Part model, mm, in its own coordinate system. A direction names the side the tool comes from. Round coordinates to 2 decimals unless told otherwise and drop trailing zeros. Loops run counter-clockwise (first coordinate to the right, second up) from the corner with the lowest first, then second, coordinate; pieces in that order, holes last.
Autodesk Inventor part; units mm, degrees
ref_plane "Start Plane" through (0, 0, 0) normal (1, 0, 0) x (0, 1, 0)
ref_plane "XZ Plane" through (0, 0, 0) normal (0, 1, 0) x (-1, 0, 0)
ref_plane "XY Plane" through (0, 0, 0) normal (0, 0, 1) x (1, 0, 0)
sketch "Main Sketch" plane through (0, 0, 0) normal (0, 0, 1) x (1, 0, 0)
  line L0 (0, 0) -> (210, 0)
  line L1 (0, 0) -> (0, 15)
  line L2 (0, 15) -> (40, 15)
  line L3 (40, 15) -> (40, 20)
  line L4 (90, 20) -> (90, 15)
  line L5 (40, 20) -> (90, 20)
  line L6 (210, 15) -> (210, 0)
  line L7 (90, 15) -> (210, 15)
  dimension "d3" = 30
  dimension "d4" = 40
  dimension "d5" = 30
revolve "Revolution1" add sketch "Main Sketch" angle 360 about axis through (0, 0, 0) along (1, 0, 0)
chamfer "Chamfer3" distance 2 angle 45 1 edges at (40, -15, 0) measured on face at (26.6667, 14.8058, -2.4062)
chamfer "Chamfer1" distance 0.5 angle 45 1 edges at (0, -15, 0) measured on face at (25.3333, 14.9514, -1.207)
chamfer "Chamfer2" distance 2 angle 45 1 edges at (90, -15, 0) measured on face at (170, 14.9514, -1.207)
equation "\"Length\" = 210"
properties part number "Shaft" material "Steel"
1) Slice it at C-C, the plane x = 53.5. Give the cut face in (y, z).
Values:
outline: circle Ø40 at (0, 0)
2) Tool access for faces 1 (the face through (40, -9, -15)), 2 (the face through (210, 0, 0)), 3 (the face through (90, -9, -15)): list every direction of +Z, -Z, +X, -X, +Y, -Y with a clear straight run to the whole face (end or side of a thin tool).
Values:
face 1: -X
face 2: +Z, -Z, +X, +Y, -Y
face 3: +X
3) Wall check: line 1 along Y through (x, z) = (83, 1); line 2 along X through (y, z) = (-8.5, -18); line 3 along Y through (x, z) = (177.5, -0.5). Give the ranges that are in metal, low to high.
Values:
line 1: y = -19.97 to 19.97
line 2: x = 40 to 90
line 3: y = -14.99 to 14.99
4) Slice it at B-B, the plane x = 96.5. Give the cut face in (y, z).
Values:
outline: circle Ø30 at (0, 0)
5) Drop flat-ended pins along their axis: pin 1 Ø12 at (x, z) = (84.5, -12) entering from -Y; pin 2 Ø6 at (x, y) = (99, -5.5) entering from +Z; pin 3 Ø1.5 at (x, y) = (50.5, -4) entering from +Z. Give the stop position or say it passes through.
Values:
pin 1: stops at y = -19.08
pin 2: stops at z = 14.79
pin 3: stops at z = 19.73
6) Slice it at A-A, the plane y = 0. Give the cut face in (x, z), then the cut area to 3 significant figures.
Values:
outline: (0, -14.5) - (0.5, -15) - (38, -15) - (40, -17) - (40, -20) - (90, -20) - (90, -17) - (92, -15) - (210, -15) - (210, 15) - (92, 15) - (90, 17) - (90, 20) - (40, 20) - (40, 17) - (38, 15) - (0.5, 15) - (0, 14.5) - close
area: 6,810 mm2
